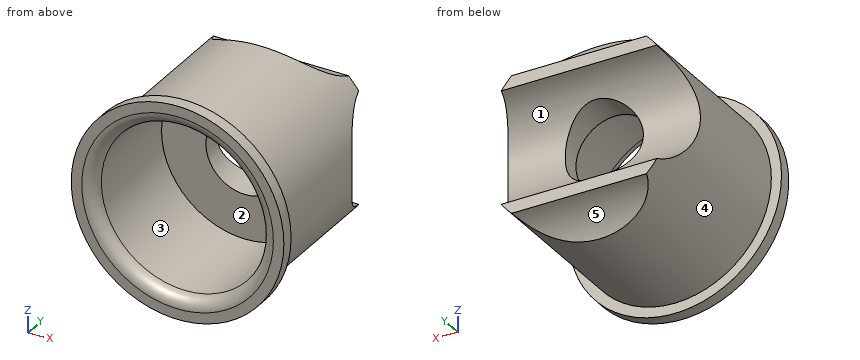
```python
from build123d import *

# Parameters (mm, degrees)
SKETCH1_R               = 8.636
BOSS_EXTRUDE1_DEPTH     = 14.2875
SKETCH5_R               = 4.7625
CUT_EXTRUDE4_DEPTH      = 9.636
CUT_EXTRUDE4_DEPTH_BACK = 9.636
SKETCH2_OUTSIDE_W       = 24.932
SKETCH2_OUTSIDE_H       = 24.932
SKETCH2_OUTSIDE_R       = 7.8105
CUT_EXTRUDE1_DEPTH      = 13.2875
SKETCH4_R               = 3.175
CUT_EXTRUDE3_DEPTH      = 15.2875
SKETCH3_R               = 6.7818
CUT_EXTRUDE2_DEPTH      = 9.31875
FILLET1_R               = 1


with BuildPart() as part:
    # Sketch1 → Boss-Extrude1 (new body)
    with BuildSketch(Plane(origin=(0, 0, 0), x_dir=(1, 0, 0), z_dir=(0, 1, 0))):
        Circle(SKETCH1_R)
    extrude(amount=BOSS_EXTRUDE1_DEPTH)

    # Sketch5 → Cut-Extrude4 (cut, two sides)
    with BuildSketch(Plane(origin=(0, 0, 0), x_dir=(0, 0, -1), z_dir=(1, 0, 0))) as cut_extrude4_sk:
        with Locations((0, 15.5575)):
            Circle(SKETCH5_R)
        with Locations((-10.16, 15.5575)):
            Circle(SKETCH5_R)
        with Locations((10.16, 15.5575)):
            Circle(SKETCH5_R)
    extrude(amount=CUT_EXTRUDE4_DEPTH, mode=Mode.SUBTRACT)
    extrude(cut_extrude4_sk.sketch, amount=-CUT_EXTRUDE4_DEPTH_BACK, mode=Mode.SUBTRACT)

    # Sketch2 outside → Cut-Extrude1 (cut)
    with BuildSketch(Plane(origin=(0, 14.2875, 0), x_dir=(1, 0, 0), z_dir=(0, 1, 0))):
        Rectangle(SKETCH2_OUTSIDE_W, SKETCH2_OUTSIDE_H)
        Circle(SKETCH2_OUTSIDE_R, mode=Mode.SUBTRACT)
    extrude(amount=-CUT_EXTRUDE1_DEPTH, mode=Mode.SUBTRACT)

    # Sketch4 → Cut-Extrude3 (cut, through all)
    with BuildSketch(Plane(origin=(0, 14.2875, 0), x_dir=(1, 0, 0), z_dir=(0, 1, 0))):
        Circle(SKETCH4_R)
    extrude(amount=-CUT_EXTRUDE3_DEPTH, mode=Mode.SUBTRACT)

    # Sketch3 → Cut-Extrude2 (cut)
    with BuildSketch(Plane.XZ):
        Circle(SKETCH3_R)
    extrude(amount=-CUT_EXTRUDE2_DEPTH, mode=Mode.SUBTRACT)

    # Fillet1
    fillet1_edges = [part.edges().sort_by_distance(p)[0] for p in [
        (-6.7818, 0, 0),
    ]]
    fillet(fillet1_edges, radius=FILLET1_R)


solid = part.part
```
Work out the finished part from the listing and answer in its coordinate system (mm). Face numbers are marked on the shaded views. A direction names the side the tool comes from. Coordinates: 2 decimals unless noted, no trailing zeros. Write each loop counter-clockwise with the first axis right and the second up, starting at its lowest first coordinate (ties: lowest second). Pieces come first, ordered by that corner, then holes.
Q1. Which of the six approach directions +Z, -Z, +X, -X, +Y, -Y give full straight-line access (tool end or side, diameter ignored) to the marked faces 1 and 2?
Q2. Determine the mould class of the marked faces 3, 4 and 5 for opening direction X: released by +X, released by -X, zero draft, split by the parting line, or undercut.
Q3. Find the intervals of material crossed by line 1 (Z direction, x = 0, y = 10.6) (1 decimal); line 2 (Z direction, x = 0, y = 4), in increasing order.
Q4. A cutting plane is placed at A-A, the plane z = 0. Give the vertices of the cut face in (x, y) (1 decimal), then the cut area to 3 significant figures.
Q5. Each of these flat-tipped pins is pushed along its axis until it touches: pin 1 Ø1.5 at (x, y) = (3.5, 5) entering from +Z; pin 2 Ø2 at (x, y) = (5, 10.5) entering from -Z; pin 3 Ø5 at (x, z) = (-2, -3.5) entering from -Y; pin 4 Ø5 at (x, z) = (0, 0) entering from -Y. Where does it stop, or does it pass through?
Q6. A cutting plane is placed at C-C, the plane y = 2.5. Give the vertices of the cut face in (x, z), then the cut area to 3 significant figures.
Q7. A cutting plane is placed at B-B, the plane x = 0. Give the vertices of the cut face in (y, z) (1 decimal).
Findings below:
1. face 1: +X, -X, +Y
1. face 2: -Y
2. face 3: undercut
2. face 4: split by the parting line
2. face 5: zero draft
3. line 1: z = -7.8 to -3.2, 3.2 to 7.8
3. line 2: z = -7.81 to -6.78, 6.78 to 7.81
4. outline: (-8.6, 0) - (-7.8, 0) arc R1 ccw to (-6.8, 1) - (-6.8, 9.3) - (-3.2, 9.3) - (-3.2, 10.8) - (-7.8, 10.8) - (-7.8, 1) - (-8.6, 1) - close; (3.2, 9.3) - (6.8, 9.3) - (6.8, 1) arc R1 ccw to (7.8, 0) - (8.6, 0) - (8.6, 1) - (7.8, 1) - (7.8, 10.8) - (3.2, 10.8) - close
4. area: 34.1 mm2
5. pin 1: stops at z = 7.31
5. pin 2: stops at z = -6.71
5. pin 3: stops at y = 9.32
5. pin 4: passes through
6. outline: circle Ø15.62 at (0, 0); hole circle Ø13.56 at (0, 0)
6. area: 47.2 mm2
7. outline: (0, -8.6) - (1, -8.6) - (1, -7.8) - (11.4, -7.8) arc R4.8 cw to (14.3, -5.6) - (14.3, -4.6) arc R4.8 cw to (12, -3.2) - (9.3, -3.2) - (9.3, -6.8) - (1, -6.8) arc R1 ccw to (0, -7.8) - close; (0, 7.8) arc R1 ccw to (1, 6.8) - (9.3, 6.8) - (9.3, 3.2) - (12, 3.2) arc R4.8 cw to (14.3, 4.6) - (14.3, 5.6) arc R4.8 cw to (11.4, 7.8) - (1, 7.8) - (1, 8.6) - (0, 8.6) - close
